Model file for the job. Use its own axes, mm. Give positions to 0.01 mm unless a question says otherwise; leave off trailing zeros. Write each loop counter-clockwise with the first axis right and the second up, starting at its lowest first coordinate (ties: lowest second). Pieces come first, ordered by that corner, then holes.
```python
from build123d import *

# Parameters (mm, degrees)
SKETCH1_W           = 429.48
SKETCH1_H           = 25.4
SKETCH1_R           = 3.175
BOSS_EXTRUDE1_DEPTH = 25.4
CUT_EXTRUDE1_REACH  = 432.98
SKETCH2_W           = 19.05
SKETCH2_H           = 19.05
SKETCH4_W           = 25.4
SKETCH4_H           = 19.05
CUT_EXTRUDE2_DEPTH  = 38.1
FILLET1_R           = 20


with BuildPart() as part:
    # Sketch1 → Boss-Extrude1 (new body)
    with BuildSketch(Plane(origin=(0, 0, 0), x_dir=(1, 0, 0), z_dir=(0, 1, 0))):
        with Locations((214.74, -12.7)):
            Rectangle(SKETCH1_W, SKETCH1_H)
        with Locations(Location((214.74, -12.7, 0), (0, 0, 270))):
            Circle(SKETCH1_R, mode=Mode.SUBTRACT)
        with Locations(Location((15.76, -12.7, 0), (0, 0, 270))):
            Circle(SKETCH1_R, mode=Mode.SUBTRACT)
        with Locations(Location((413.72, -12.7, 0), (0, 0, 90))):
            Circle(SKETCH1_R, mode=Mode.SUBTRACT)
    extrude(amount=BOSS_EXTRUDE1_DEPTH)

    # Cut-Extrude1: up to this face of the body (flat: up to its plane)
    cut_extrude1_end = Plane(part.part.faces().sort_by_distance((429.48, 12.7, 12.7))[0])
    # Sketch2 → Cut-Extrude1 (cut, up to the picked face)
    with BuildSketch(Plane.ZY, mode=Mode.PRIVATE) as cut_extrude1_sk1:
        with Locations((12.7, 12.7)):
            Rectangle(SKETCH2_W, SKETCH2_H)
    cut_extrude1_tool1 = split(extrude(cut_extrude1_sk1.sketch, amount=-CUT_EXTRUDE1_REACH, mode=Mode.PRIVATE), bisect_by=cut_extrude1_end, keep=Keep.BOTH, mode=Mode.PRIVATE)
    add(cut_extrude1_tool1.solids().sort_by(Axis((0, 12.7, 12.7), (1, 0, 0)))[0], mode=Mode.SUBTRACT)

    # Sketch4 → Cut-Extrude2 (cut)
    with BuildSketch(Plane.ZY):
        with Locations((12.7, 12.7)):
            Rectangle(SKETCH4_W, SKETCH4_H)
    cut_extrude2 = extrude(amount=-CUT_EXTRUDE2_DEPTH, mode=Mode.SUBTRACT)

    # Mirror1: Cut-Extrude2 across plane
    add(cut_extrude2.mirror(Plane.ZY.offset(-214.74)), mode=Mode.SUBTRACT)

    # Fillet1
    # the kernel refuses this fillet: 20 mm, written as the material it takes off along each edge
    with BuildSketch(Plane(origin=(429.48, -50, 0), x_dir=(-1, 0, 0), z_dir=(0, 1, 0)), Plane(origin=(429.48, -27.775, 0), x_dir=(-1, 0, 0), z_dir=(0, 1, 0)), Plane(origin=(0, -27.775, 25.4), x_dir=(1, 0, 0), z_dir=(0, 1, 0))) as fillet1_piece_1:
        with BuildLine():
            CenterArc((FILLET1_R, FILLET1_R), FILLET1_R, 180, 90)
            Line((0, FILLET1_R), (0, 0))
            Line((0, 0), (FILLET1_R, 0))
        make_face()
    extrude(amount=103.175, mode=Mode.SUBTRACT)
    with BuildSketch(Plane(origin=(429.48, -50, 25.4), x_dir=(-1, 0, 0), z_dir=(0, 1, 0)), Plane(origin=(429.48, -27.775, 25.4), x_dir=(-1, 0, 0), z_dir=(0, 1, 0)), Plane(origin=(0, -50, 25.4), x_dir=(0, 0, -1), z_dir=(0, 1, 0)), Plane(origin=(0, -50, 0), x_dir=(1, 0, 0), z_dir=(0, 1, 0)), Plane(origin=(0, -27.775, 0), x_dir=(1, 0, 0), z_dir=(0, 1, 0))) as fillet1_piece_2:
        with BuildLine():
            CenterArc((FILLET1_R, -FILLET1_R), FILLET1_R, 90, 90)
            Line((0, -FILLET1_R), (0, 0))
            Line((0, 0), (FILLET1_R, 0))
        make_face()
    extrude(amount=103.175, mode=Mode.SUBTRACT)


solid = part.part
```
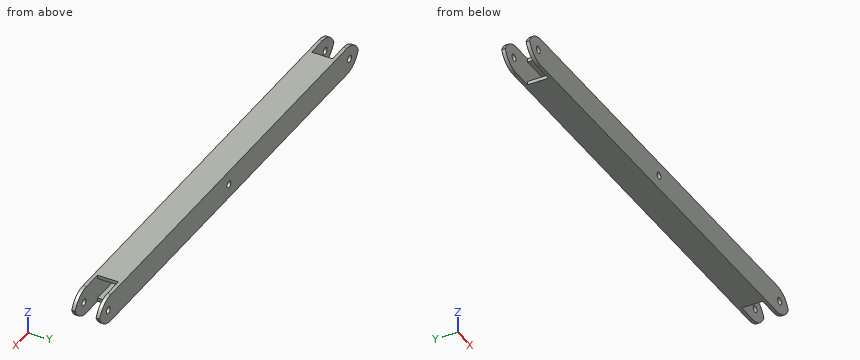
1. Pin check, flat tips, straight feed: P1, Ø1, axis at y = 13.5, z = 2, coming from the -X side; P2, Ø8, axis at y = 2.5, z = 17, coming from the +X side; P3, Ø3.5, axis at y = 12.5, z = 2, coming from the +X side; P4, Ø5.5, axis at x = 413.72, z = 12.7, coming from the +Y side. Stop position of each tip, or through.
Calculated:
P1: stops at x = 38.1
P2: stops at x = 427.98
P3: stops at x = 391.38
P4: passes through
2. Slice it at B-B, the plane y = 8.5. Write the cut outline in (x, z) (3 decimals).
Calculated:
outline: (38.1, 0) - (391.38, 0) - (391.38, 3.175) - (38.1, 3.175) - close; (38.1, 22.225) - (391.38, 22.225) - (391.38, 25.4) - (38.1, 25.4) - close
3. Probe probe 1 along Y at (x, z) = (409, 13.25) (3 decimals); probe 2 along X at (y, z) = (8.5, 2.5). List the from-to ranges inside material, lowest first.
Calculated:
probe 1: y = 0 to 3.175, 22.225 to 25.4
probe 2: x = 38.1 to 391.38
4. Slice it at A-A, the plane x = 201. Write the cut outline in (y, z) (3 decimals), and give its area (3 significant figures).
Calculated:
outline: (0, 0) - (25.4, 0) - (25.4, 25.4) - (0, 25.4) - close; hole (3.175, 3.175) - (22.225, 3.175) - (22.225, 22.225) - (3.175, 22.225) - close
area: 282 mm2
